Could you check a few things on this model? Use its own coordinates, in mm. A direction names the side the tool comes from. Give positions to 0.01 mm unless a question says otherwise; leave off trailing zeros. Order: outer loops, then holes, each group sorted by start corner. A loop starts at its lowest first (then second) coordinate and runs counter-clockwise, first axis right, second up.
(1) Imagine slicing it at C-C, the plane z = 20.75. Write out the boundary of the cut face in (x, y), then the cut area to 3 significant figures.
(2) Will these pins go through, and if not, where does the flat tip stop? pin 1 (3 mm diameter, centred on y = 6.5, z = 30.5, fed in from -X); pin 2 (3 mm diameter, centred on y = 5, z = 30, fed in from +X); pin 3 (3 mm diameter, centred on x = 3.5, z = 32.5, fed in from +Y).
(3) If we mould it in two halves opening along Z, with no side actions, what happens to faces 4 (the flat face through (3.2, -0.2, 34.673)), 5 (the flat face through (3, 5, 37.873)), 6 (the flat face through (5.4, 11, 31))? For each: released by +Z, released by -Z, zero draft, split by the parting line, or undercut.
(4) On a 3-axis mill with a long thin cutter (end or side, diameter ignored), from which of +Z, -Z, +X, -X, +Y, -Y can I reach the whole of each face in a straight line? I mean faces 1 (the flat face through (3, -2, 19.773)), 2 (the flat face through (1.87, 11, 31)), 3 (the flat face through (3, -2, 35.913)). Say none if no direction works.
(5) Imagine slicing it at D-D, the plane y = 1.5. Write out the boundary of the cut face in (x, z).
(6) Imagine slicing it at B-B, the plane x = 0.5. Write out the boundary of the cut face in (y, z) (3 decimals), then the cut area to 3 significant figures.
(7) If I drill on probe 1 along Z at (x, y) = (3.5, -1.25); probe 2 along Y at (x, z) = (4.5, 33); probe 3 along X at (y, z) = (1, 37), over which ranges is the centre line in solid material (lowest first)?
(8) Imagine slicing it at A-A, the plane y = -2.5. Write out the boundary of the cut face in (x, z).
from build123d import *

# Parameters (mm, degrees)
SKETCH1_R           = 1.275
BOSS_EXTRUDE1_DEPTH = 6.5
SKETCH2_W           = 3.53
SKETCH2_H           = 1.96
BOSS_EXTRUDE2_DEPTH = 1.2
FILLET1_R           = 0.7
SKETCH3_W           = 3.2
SKETCH3_H           = 0.56
SKETCH3_H_2         = 0.5
BOSS_EXTRUDE3_DEPTH = 0.9
SKETCH4_W           = 1.2
SKETCH4_H           = 0.56
SKETCH4_H_2         = 0.5
BOSS_EXTRUDE4_DEPTH = 3.47
FILLET2_R           = 0.59
EXTRUDE_START       = -1.5
EXTRUDE_1_DEPTH     = 4
FILLET_1_R          = 0.5
EXTRUDE1_DEPTH      = 0.25
EXTRUDE2_START      = -6.5
EXTRUDE2_DEPTH      = 0.25


with BuildPart() as part:
    # Sketch1 → Boss-Extrude1 (new body)
    with BuildSketch(Plane(origin=(0, 0, 0), x_dir=(0, 0, -1), z_dir=(1, 0, 0))):
        with BuildLine():
            Line((-37.373122581, 0), (-34.673122581, 0))
            Line((-34.673122581, 0), (-34.673122581, -0.45))
            Line((-34.673122581, -0.45), (-30.873122581, -0.45))
            Line((-30.873122581, -0.45), (-30.873122581, 0))
            Line((-30.873122581, 0), (-24.973122581, 0))
            Line((-24.973122581, 0), (-24.973122581, -0.45))
            Line((-24.973122581, -0.45), (-21.173122581, -0.45))
            Line((-21.173122581, -0.45), (-21.173122581, 0))
            Line((-21.173122581, 0), (-18.673122581, 0))
            ThreePointArc((-18.673122581, 0), (-18.31956919, 0.146446609), (-18.173122581, 0.5))
            Line((-18.173122581, 0.5), (-18.173122581, 9.02))
            ThreePointArc((-18.173122581, 9.02), (-18.31956919, 9.373553391), (-18.673122581, 9.52))
            Line((-18.673122581, 9.52), (-28.173122581, 9.52))
            Line((-28.173122581, 9.52), (-28.173122581, 10.16))
            Line((-28.173122581, 10.16), (-37.373122581, 10.16))
            ThreePointArc((-37.373122581, 10.16), (-37.726675972, 10.013553391), (-37.873122581, 9.66))
            Line((-37.873122581, 9.66), (-37.873122581, 0.5))
            ThreePointArc((-37.873122581, 0.5), (-37.726675972, 0.146446609), (-37.373122581, 0))
        make_face()
        with Locations((-32.773122581, 2.525)):
            Circle(SKETCH1_R, mode=Mode.SUBTRACT)
        with Locations((-23.073122581, 2.525)):
            Circle(SKETCH1_R, mode=Mode.SUBTRACT)
    extrude(amount=BOSS_EXTRUDE1_DEPTH)

    # Sketch2 → Boss-Extrude2 (add)
    with BuildSketch(Plane(origin=(0, 10.16, 0), x_dir=(1, 0, 0), z_dir=(0, 1, 0))):
        with Locations((3.635, -30.693122581)):
            Rectangle(SKETCH2_W, SKETCH2_H)
    extrude(amount=BOSS_EXTRUDE2_DEPTH)

    # Fillet1
    fillet1_edges = [part.edges().sort_by_distance(p)[0] for p in [
        (3.635, 11.36, 31.673122581),
        (3.635, 11.36, 29.713122581),
    ]]
    fillet(fillet1_edges, radius=FILLET1_R)

    # Sketch3 → Boss-Extrude3 (add)
    with BuildSketch(Plane(origin=(0, 0, 0), x_dir=(-1, 0, 0), z_dir=(0, -1, 0))):
        with Locations((-3.25, -36.193122581)):
            Rectangle(SKETCH3_W, SKETCH3_H)
        with Locations((-3.25, -27.223122581)):
            Rectangle(SKETCH3_W, SKETCH3_H_2)
        with Locations((-3.25, -20.023122581)):
            Rectangle(SKETCH3_W, SKETCH3_H_2)
    extrude(amount=BOSS_EXTRUDE3_DEPTH)

    # Sketch4 → Boss-Extrude4 (add)
    with BuildSketch(Plane(origin=(0, -0.9, 0), x_dir=(-1, 0, 0), z_dir=(0, -1, 0))):
        with Locations((-3.25, -36.193122581)):
            Rectangle(SKETCH4_W, SKETCH4_H)
        with Locations((-3.25, -27.223122581)):
            Rectangle(SKETCH4_W, SKETCH4_H_2)
        with Locations((-3.25, -20.023122581)):
            Rectangle(SKETCH4_W, SKETCH4_H_2)
    extrude(amount=BOSS_EXTRUDE4_DEPTH)

    # Fillet2
    fillet2_edges = [part.edges().sort_by_distance(p)[0] for p in [
        (2.65, -4.37, 36.193122581),
        (3.85, -4.37, 36.193122581),
        (2.65, -4.37, 27.223122581),
        (3.85, -4.37, 27.223122581),
        (3.85, -4.37, 20.023122581),
        (2.65, -4.37, 20.023122581),
    ]]
    fillet(fillet2_edges, radius=FILLET2_R)

    # Эскиз1 → Бобышка-Вытянуть1 (add)
    with BuildSketch(Plane(origin=(6.5, 0, 0), x_dir=(0, 0, -1), z_dir=(1, 0, 0)).offset(EXTRUDE_START)):
        Polygon((-34.851945428, 10.16), (-34.851945428, 10.976764044), (-18.550578779, 12.570949573), (-18.570044834, 12.77), (-35.033122581, 11.16), (-35.033122581, 10.16), align=None)
    extrude(amount=-EXTRUDE_1_DEPTH)

    # Скругление1
    fillet_1_edges = [part.edges().sort_by_distance(p)[0] for p in [
        (3, 11.16, 35.033122581),
        (3, 10.976764044, 34.851945428),
    ]]
    fillet(fillet_1_edges, radius=FILLET_1_R)

    # Sketch6 → Extrude1 (cut)
    with BuildSketch(Plane(origin=(6.5, 0, 0), x_dir=(0, 0, -1), z_dir=(1, 0, 0))):
        with BuildLine():
            Line((-34.673122581, 0), (-34.673122581, 2.525))
            ThreePointArc((-34.673122581, 2.525), (-32.773122581, 4.425), (-30.873122581, 2.525))
            Line((-30.873122581, 2.525), (-30.873122581, 0))
            Line((-30.873122581, 0), (-24.973122581, 0))
            Line((-24.973122581, 0), (-24.973122581, 2.525))
            ThreePointArc((-24.973122581, 2.525), (-23.073122581, 4.425), (-21.173122581, 2.525))
            Line((-21.173122581, 2.525), (-21.173122581, 0))
            Line((-21.173122581, 0), (-18.673122581, 0))
            ThreePointArc((-18.673122581, 0), (-18.31956919, 0.146446609), (-18.173122581, 0.5))
            Line((-18.173122581, 0.5), (-18.173122581, 9.02))
            ThreePointArc((-18.173122581, 9.02), (-18.31956919, 9.373553391), (-18.673122581, 9.52))
            Line((-18.673122581, 9.52), (-28.173122581, 9.52))
            Line((-28.173122581, 9.52), (-28.173122581, 10.16))
            Line((-28.173122581, 10.16), (-37.373122581, 10.16))
            ThreePointArc((-37.373122581, 10.16), (-37.726675972, 10.013553391), (-37.873122581, 9.66))
            Line((-37.873122581, 9.66), (-37.873122581, 0.5))
            ThreePointArc((-37.873122581, 0.5), (-37.726675972, 0.146446609), (-37.373122581, 0))
            Line((-37.373122581, 0), (-34.673122581, 0))
        make_face()
    extrude(amount=-EXTRUDE1_DEPTH, mode=Mode.SUBTRACT)

    # Sketch → Extrude2 (cut)
    with BuildSketch(Plane(origin=(6.5, 0, 0), x_dir=(0, 0, -1), z_dir=(1, 0, 0)).offset(EXTRUDE2_START)):
        with BuildLine():
            Line((-34.673122581, 0), (-34.673122581, 2.525))
            ThreePointArc((-34.673122581, 2.525), (-32.773122581, 4.425), (-30.873122581, 2.525))
            Line((-30.873122581, 2.525), (-30.873122581, 0))
            Line((-30.873122581, 0), (-24.973122581, 0))
            Line((-24.973122581, 0), (-24.973122581, 2.525))
            ThreePointArc((-24.973122581, 2.525), (-23.073122581, 4.425), (-21.173122581, 2.525))
            Line((-21.173122581, 2.525), (-21.173122581, 0))
            Line((-21.173122581, 0), (-18.673122581, 0))
            ThreePointArc((-18.673122581, 0), (-18.31956919, 0.146446609), (-18.173122581, 0.5))
            Line((-18.173122581, 0.5), (-18.173122581, 9.02))
            ThreePointArc((-18.173122581, 9.02), (-18.31956919, 9.373553391), (-18.673122581, 9.52))
            Line((-18.673122581, 9.52), (-28.173122581, 9.52))
            Line((-28.173122581, 9.52), (-28.173122581, 10.16))
            Line((-28.173122581, 10.16), (-37.373122581, 10.16))
            ThreePointArc((-37.373122581, 10.16), (-37.726675972, 10.013553391), (-37.873122581, 9.66))
            Line((-37.873122581, 9.66), (-37.873122581, 0.5))
            ThreePointArc((-37.873122581, 0.5), (-37.726675972, 0.146446609), (-37.373122581, 0))
            Line((-37.373122581, 0), (-34.673122581, 0))
        make_face()
    extrude(amount=EXTRUDE2_DEPTH, mode=Mode.SUBTRACT)


solid = part.part
Answer block:
1. outline: (0.25, 0) - (6.25, 0) - (6.25, 9.52) - (0.25, 9.52) - close; (1, 12.36) - (5, 12.36) - (5, 12.56) - (1, 12.56) - close
1. area: 57.9 mm2
2. pin 1: stops at x = 0.25
2. pin 2: stops at x = 6.25
2. pin 3: stops at y = 11.55
3. face 4: undercut
3. face 5: released by +Z
3. face 6: zero draft
4. face 1: -Z, +X, -X, -Y
4. face 2: -Z, -X
4. face 3: +X, -X, -Y
5. outline: (0, 21.17) - (0.25, 21.17) - (0.25, 18.17) - (6.25, 18.17) - (6.25, 21.17) - (6.5, 21.17) - (6.5, 22.31) - (0, 22.31) - close; (0, 23.83) - (6.5, 23.83) - (6.5, 24.97) - (6.25, 24.97) - (6.25, 30.87) - (6.5, 30.87) - (6.5, 32.01) - (0, 32.01) - (0, 30.87) - (0.25, 30.87) - (0.25, 24.97) - (0, 24.97) - close; (0, 33.53) - (6.5, 33.53) - (6.5, 34.67) - (6.25, 34.67) - (6.25, 37.87) - (0.25, 37.87) - (0.25, 34.67) - (0, 34.67) - close
6. outline: (-0.45, 21.173) - (0, 21.173) - (0, 18.673) arc R0.5 ccw to (0.5, 18.173) - (9.02, 18.173) arc R0.5 ccw to (9.52, 18.673) - (9.52, 28.173) - (10.16, 28.173) - (10.16, 37.373) arc R0.5 ccw to (9.66, 37.873) - (0.5, 37.873) arc R0.5 ccw to (0, 37.373) - (0, 34.673) - (-0.45, 34.673) - (-0.45, 30.873) - (0, 30.873) - (0, 24.973) - (-0.45, 24.973) - close; hole circle Ø2.55 at (2.525, 23.073); hole circle Ø2.55 at (2.525, 32.773)
6. area: 187 mm2
7. probe 1: z = 19.77 to 20.27, 26.97 to 27.47, 35.91 to 36.47
7. probe 2: y = -0.45 to 1.27, 3.78 to 10.16, 11.16 to 11.36
7. probe 3: x = 0.25 to 6.25
8. outline: (2.65, 19.77) - (3.85, 19.77) - (3.85, 20.27) - (2.65, 20.27) - close; (2.65, 26.97) - (3.85, 26.97) - (3.85, 27.47) - (2.65, 27.47) - close; (2.65, 35.91) - (3.85, 35.91) - (3.85, 36.47) - (2.65, 36.47) - close
